CAD build for the part. Positions are in the model's coordinates, mm. A direction names the side the tool comes from. Coordinates: 2 decimals unless noted, no trailing zeros. Order: outer loops, then holes, each group sorted by start corner. A loop starts at its lowest first (then second) coordinate and runs counter-clockwise, first axis right, second up. Notation, with made-up numbers: (-30, 37) -> (17, 37) arc R18 ccw to (17, 45) -> close; hole circle Ø1 at (39.5, 56). An arc over 180 degrees is marked (long way). Use one line per item in the form item = value. Start each with the question number.
from build123d import *

# Parameters (mm, degrees)
SKETCH1_W                      = 65
SKETCH1_H                      = 8.5
BOSS_EXTRUDE1_DEPTH            = 120
F_6_0MM_DOWEL_HOLE1_AT_2_COUNT = 2
F_6_0MM_DOWEL_HOLE1_AT_2_PITCH = 24.5
F_6_0MM_DOWEL_HOLE1_AT_3_COUNT = 2
F_6_0MM_DOWEL_HOLE1_AT_3_PITCH = 49
F_6_0MM_DOWEL_HOLE2_AT_2_COUNT = 2
F_6_0MM_DOWEL_HOLE2_AT_2_PITCH = 100
CUT_EXTRUDE1_DEPTH             = 9.5
F_3_0MM_DOWEL_HOLE1_D          = 3.5


with BuildPart() as part:
    # Sketch1 → Boss-Extrude1 (new body)
    with BuildSketch(Plane(origin=(0, 0, 0), x_dir=(0, 0, -1), z_dir=(1, 0, 0))):
        Rectangle(SKETCH1_W, SKETCH1_H)
    extrude(amount=BOSS_EXTRUDE1_DEPTH)

    # Sketch3 → Ø6.0mm Dowel Hole1 (revolve, cut)
    with BuildSketch(Plane(origin=(120, 0, 24.5), x_dir=(0, 0, -1), z_dir=(0, 1, 0))):
        Polygon((0, 0), (0, 11.802581857), (3, 10), (3, 0), align=None)
    f_6_0mm_dowel_hole1 = revolve(axis=Axis((126.35, 0, 24.5), (-1, 0, 0)), mode=Mode.SUBTRACT)

    # Ø6.0mm Dowel Hole1 at 2: Ø6.0mm Dowel Hole1 ×2
    with Locations(*[(0, 0, -i * F_6_0MM_DOWEL_HOLE1_AT_2_PITCH) for i in range(1, F_6_0MM_DOWEL_HOLE1_AT_2_COUNT)]):
        add(f_6_0mm_dowel_hole1, mode=Mode.SUBTRACT)

    # Ø6.0mm Dowel Hole1 at 3: Ø6.0mm Dowel Hole1 ×2
    with Locations(*[(0, 0, -i * F_6_0MM_DOWEL_HOLE1_AT_3_PITCH) for i in range(1, F_6_0MM_DOWEL_HOLE1_AT_3_COUNT)]):
        add(f_6_0mm_dowel_hole1, mode=Mode.SUBTRACT)

    # Mirror1: Ø6.0mm Dowel Hole1 across plane
    add(f_6_0mm_dowel_hole1.mirror(Plane(origin=(60, 0, 0), x_dir=(0, 0, 1), z_dir=(1, 0, 0))), mode=Mode.SUBTRACT)

    # Mirror1 copy 1 sketch → Mirror1 copy 1 (revolve, cut)
    with BuildSketch(Plane(origin=(0, 0, 0), x_dir=(0, 0, -1), z_dir=(0, 1, 0))):
        Polygon((0, 0), (0, -11.802581857), (3, -10), (3, 0), align=None)
    revolve(axis=Axis((-6.35, 0, 0), (-1, 0, 0)), mode=Mode.SUBTRACT)

    # Mirror1 copy 2 sketch → Mirror1 copy 2 (revolve, cut)
    with BuildSketch(Plane(origin=(0, 0, -24.5), x_dir=(0, 0, -1), z_dir=(0, 1, 0))):
        Polygon((0, 0), (0, -11.802581857), (3, -10), (3, 0), align=None)
    revolve(axis=Axis((-6.35, 0, -24.5), (-1, 0, 0)), mode=Mode.SUBTRACT)

    # Sketch5 → Ø6.0mm Dowel Hole2 (revolve, cut)
    with BuildSketch(Plane(origin=(110, 0, -32.5), x_dir=(0, 1, 0), z_dir=(1, 0, 0))):
        Polygon((0, 0), (0, 9.802581857), (3, 8), (3, 0), align=None)
    f_6_0mm_dowel_hole2 = revolve(axis=Axis((110, 0, -38.85), (0, 0, 1)), mode=Mode.SUBTRACT)

    # Ø6.0mm Dowel Hole2 at 2: Ø6.0mm Dowel Hole2 ×2
    with Locations(*[(-i * F_6_0MM_DOWEL_HOLE2_AT_2_PITCH, 0, 0) for i in range(1, F_6_0MM_DOWEL_HOLE2_AT_2_COUNT)]):
        add(f_6_0mm_dowel_hole2, mode=Mode.SUBTRACT)

    # Mirror2: Ø6.0mm Dowel Hole2 across plane
    add(f_6_0mm_dowel_hole2.mirror(Plane.XY), mode=Mode.SUBTRACT)

    # Mirror2 copy 1 sketch → Mirror2 copy 1 (revolve, cut)
    with BuildSketch(Plane(origin=(10, 0, 32.5), x_dir=(0, 1, 0), z_dir=(1, 0, 0))):
        Polygon((0, 0), (0, -9.802581857), (3, -8), (3, 0), align=None)
    revolve(axis=Axis((10, 0, 38.85), (0, 0, 1)), mode=Mode.SUBTRACT)

    # Sketch6 → Cut-Extrude1 (cut, through all)
    with BuildSketch(Plane(origin=(0, 4.25, 0), x_dir=(1, 0, 0), z_dir=(0, 1, 0))):
        with BuildLine():
            Line((80, -7), (80, 7))
            ThreePointArc((80, 7), (86, 13), (92, 7))
            Line((92, 7), (92, -7))
            ThreePointArc((92, -7), (86, -13), (80, -7))
        make_face()
    cut_extrude1 = extrude(amount=-CUT_EXTRUDE1_DEPTH, mode=Mode.SUBTRACT)

    # Mirror3: Cut-Extrude1 across plane
    add(cut_extrude1.mirror(Plane(origin=(60, 0, 0), x_dir=(0, 0, 1), z_dir=(1, 0, 0))), mode=Mode.SUBTRACT)

    # Ø3.0mm Dowel Hole1 (through all)
    with Locations(Plane(origin=(0, 4.25, 0), x_dir=(1, 0, 0), z_dir=(0, 1, 0))):
        with Locations((87, -17), (87, 17), (33, 17), (33, -17), (100, -24.5), (60, -24.5), (20, -24.5), (100, 24.5), (60, 24.5), (20, 24.5)):
            Hole(F_3_0MM_DOWEL_HOLE1_D / 2)


solid = part.part
1) Cut at C-C on x = 33. Give the cut face in (y, z), then the cut area to 3 significant figures.
2) Cut at D-D on y = 1.5. Count the separate pieces of the cut face and the enclosed holes in it, then the cut area to 3 significant figures.
3) Drop flat-ended pins along their axis: P1, Ø2.5, axis at y = -0.5, z = 1.5, coming from the -X side; P2, Ø3.5, axis at x = 10, y = 0, coming from the -Z side; P3, Ø3.5, axis at y = 0, z = 0, coming from the +X side. Give the stop position or say it passes through.
4) 3-axis set-ups, long thin cutter, end or side, ignore diameter. For faces 1 (the face through (115.07, -0.9, 21.64)), 2 (the face through (109.195, 0.036, 22.841)), 3 (the face through (4.93, -0.9, 21.64)), 4 (the face through (12.93, -0.65, -28.56)), 5 (the face through (28, 0, 0)): which of +Z, -Z, +X, -X, +Y, -Y reach the whole face in a straight line?
5) Probe L1, parallel to Z at x = 20, y = -2.5; L2, parallel to X at y = 0, z = 28.5; L3, parallel to Z at x = 5.25, y = 0. List the from-to ranges inside material, lowest first.
6) Cut at A-A on z = -17. Give the cut face in (x, y).
7) Two-plate mould, pull along Y, no slides. Class faces 6 (the face through (12.93, -0.65, 28.56)), 7 (the face through (59, 0, 32.5)), 8 (the face through (59, -4.25, 0)): released by +Y, released by -Y, zero draft, split by the parting line, or undercut.
8) Cut at B-B on x = 60. Give the cut face in (y, z).
Values follow:
q1.outline = (-4.25, -32.5) -> (4.25, -32.5) -> (4.25, -18.75) -> (-4.25, -18.75) -> close; (-4.25, -15.25) -> (4.25, -15.25) -> (4.25, -12.92) -> (-4.25, -12.92) -> close; (-4.25, 12.92) -> (4.25, 12.92) -> (4.25, 15.25) -> (-4.25, 15.25) -> close; (-4.25, 18.75) -> (4.25, 18.75) -> (4.25, 32.5) -> (-4.25, 32.5) -> close
q1.area = 273 mm^2
q2.separate_pieces = 5
q2.enclosed_holes = 12
q2.area = 6,680 mm^2
q3.P1 = 10.1
q3.P2 = -23.75
q3.P3 = 109.25
q4.face_1 = +X
q4.face_2 = +Z, +X
q4.face_3 = -X
q4.face_4 = -Z
q4.face_5 = +Y, -Y
q5.L1 = -32.5 to -26.25, -22.75 to 22.75, 26.25 to 32.5
q5.L2 = 0 to 7, 13 to 107, 113 to 120
q5.L3 = -32.5 to -27.5, -21.5 to -3, 3 to 21.5, 27.5 to 32.5
q6.outline = (0, -4.25) -> (31.25, -4.25) -> (31.25, 4.25) -> (0, 4.25) -> close; (34.75, -4.25) -> (85.25, -4.25) -> (85.25, 4.25) -> (34.75, 4.25) -> close; (88.75, -4.25) -> (120, -4.25) -> (120, 4.25) -> (88.75, 4.25) -> close
q7.face_6 = undercut
q7.face_7 = zero draft
q7.face_8 = released by -Y
q8.outline = (-4.25, -32.5) -> (4.25, -32.5) -> (4.25, -26.25) -> (-4.25, -26.25) -> close; (-4.25, -22.75) -> (4.25, -22.75) -> (4.25, 22.75) -> (-4.25, 22.75) -> close; (-4.25, 26.25) -> (4.25, 26.25) -> (4.25, 32.5) -> (-4.25, 32.5) -> close
